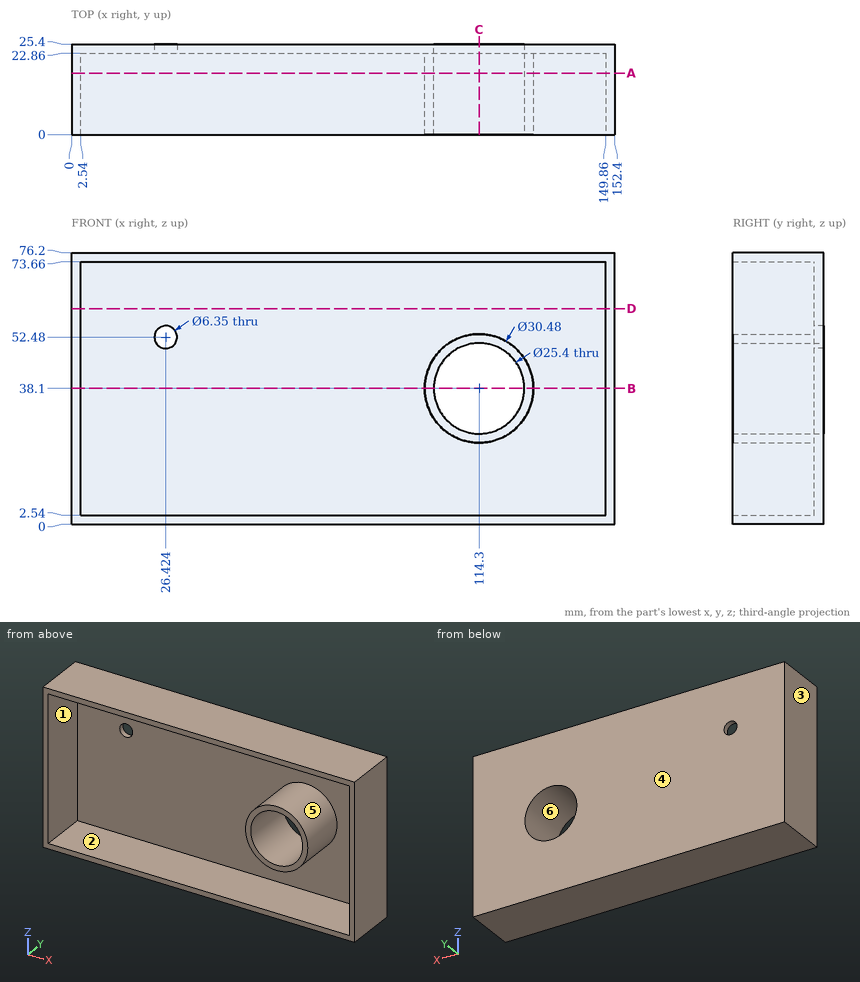
Source: three-view drawing plus pictorial views. Frame: mm from the lowest corner of the part. A direction names the side the tool comes from. Round coordinates to 2 decimals unless told otherwise and drop trailing zeros. Loops run counter-clockwise (first coordinate to the right, second up) from the corner with the lowest first, then second, coordinate; pieces in that order, holes last. Notation, with made-up numbers: M 48.5,-7.5 L 66.5,-7.5 A19 cw 66.5,23.5 Z; hole C 87.5,-10 d4. An arc over 180 degrees is marked long. Answer as CSV lines item,"result". Start each with the question number.
(1) Line query: line 1 (Z direction, x = 114.3, y = 18.75); line 2 (Z direction, x = 11.5, y = 20.5); line 3 (X direction, y = 4, z = 64.5). Output: solid intervals per line, ascending. Write a range as [from, to].
(2) Reachability of the marked faces 5 and 6 from +Z, -Z, +X, -X, +Y, -Y: full face, straight path, thin tool, end or side. Return the list, or none.
(3) First-contact query: pin 1 (12 mm diameter, centred on x = 16, z = 22, fed in from -Y). Flat tip, straight axial feed; report the tip coordinate or a pass-through.
(4) Section C-C, the plane x = 114.3. Output: boundary loops of the cut face in (y, z).
(5) Section A-A, the plane y = 17.25. Output: boundary loops of the cut face in (x, z).
(6) Section D-D, the plane z = 60.5. Output: boundary loops of the cut face in (x, y), plus the area to 3 significant figures.
(7) Section B-B, the plane z = 38.1. Output: boundary loops of the cut face in (x, y).
(8) Draft query along X for the marked faces 1, 2, 3 and 4. Return one class per face: released by +X, released by -X, zero draft, split by the parting line, or undercut.
Values found:
1,line 1,"z = [0, 2.54], [22.86, 25.4], [50.8, 53.34], [73.66, 76.2]"
1,line 2,"z = [0, 2.54], [73.66, 76.2]"
1,line 3,"x = [0, 2.54], [149.86, 152.4]"
2,face 5,"-Y"
2,face 6,"+Y, -Y"
3,pin 1,"stops at y = 22.86"
4,outline,"M 0,0 L 25.4,0 L 25.4,25.4 L 0,25.4 L 0,22.86 L 22.86,22.86 L 22.86,2.54 L 0,2.54 Z; M 0,50.8 L 25.4,50.8 L 25.4,76.2 L 0,76.2 L 0,73.66 L 22.86,73.66 L 22.86,53.34 L 0,53.34 Z"
5,outline,"M 0,0 L 152.4,0 L 152.4,76.2 L 0,76.2 Z; C 114.3,38.1 d30.48; hole M 2.54,2.54 L 149.86,2.54 L 149.86,73.66 L 2.54,73.66 Z; hole C 114.3,38.1 d25.4"
6,outline,"M 0,0 L 2.54,0 L 2.54,22.86 L 149.86,22.86 L 149.86,0 L 152.4,0 L 152.4,25.4 L 0,25.4 Z"
6,area,"503 mm²"
7,outline,"M 0,0 L 2.54,0 L 2.54,22.86 L 99.06,22.86 L 99.06,0 L 101.6,0 L 101.6,25.4 L 0,25.4 Z; M 127,0 L 129.54,0 L 129.54,22.86 L 149.86,22.86 L 149.86,0 L 152.4,0 L 152.4,25.4 L 127,25.4 Z"
8,face 1,"undercut"
8,face 2,"undercut"
8,face 3,"released by -X"
8,face 4,"zero draft"
